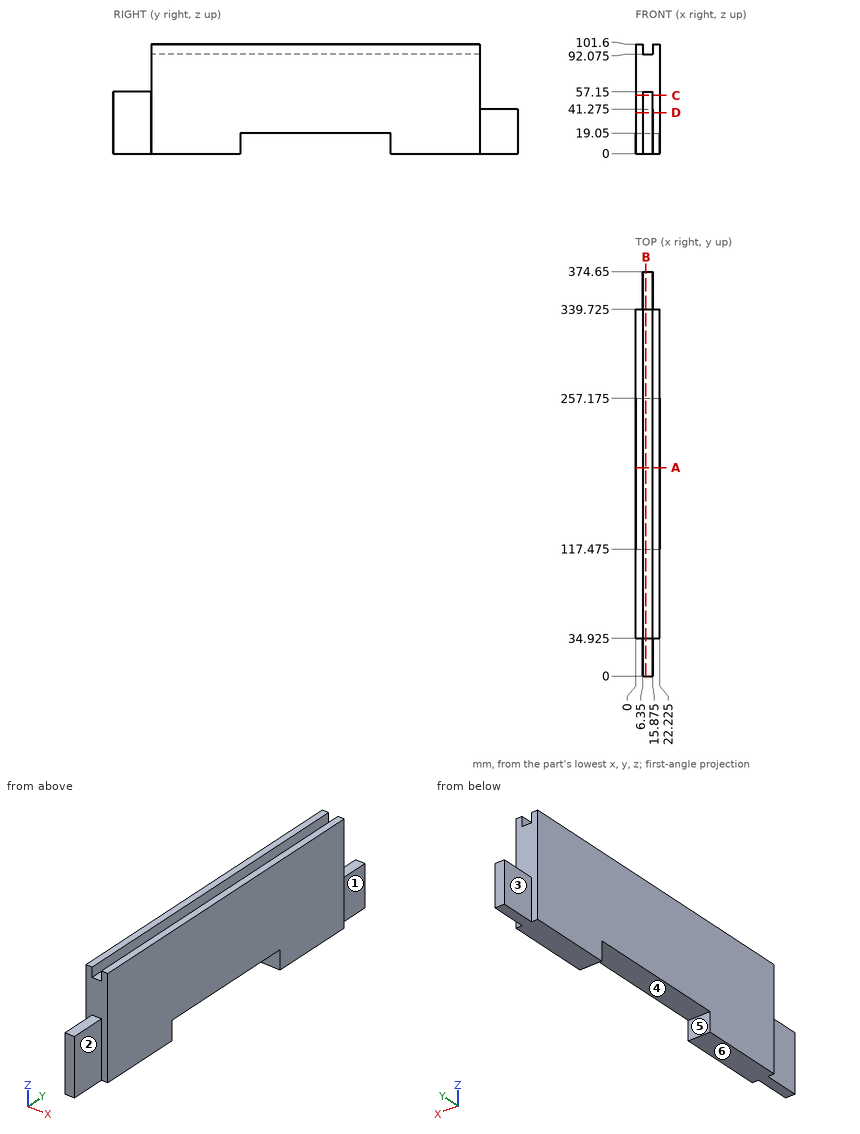
The figure shows three views and two pictorial views of one solid part (mm, origin at its lowest corner). Answer the questions. A direction names the side the tool comes from. Coordinates: 2 decimals unless noted, no trailing zeros. Order: outer loops, then holes, each group sorted by start corner. A loop starts at its lowest first (then second) coordinate and runs counter-clockwise, first axis right, second up.
Q1. A cutting plane is placed at C-C, the plane z = 54. Write down the section's boundary in (x, y) (3 decimals), and give its area (3 significant figures).
Q2. A cutting plane is placed at B-B, the plane x = 9.5. Write down the section's boundary in (y, z) (3 decimals).
Q3. A cutting plane is placed at D-D, the plane z = 38. Write down the section's boundary in (x, y) (3 decimals).
Q4. Given P1, Ø11, axis at x = 16, y = 198, coming from the -Z side; P2, Ø5, axis at x = 12, y = 250, coming from the +Z side (3 decimals); P3, Ø5, axis at x = 9.5, z = 79.5, coming from the +Y side (3 decimals), each flat-ended and moving along its own axis, determine where each tip first touches the part or whether it passes through.
Q5. Which of the six approach directions +Z, -Z, +X, -X, +Y, -Y give full straight-line access (tool end or side, diameter ignored) to the marked faces 1, 2, 3 and 4?
Q6. A cutting plane is placed at A-A, the plane y = 193. Write down the section's boundary in (x, z) (3 decimals), and give its area (3 significant figures).
Q7. Consider line 1 (Y direction, x = 9, z = 7) (3 decimals); line 2 (Y direction, x = 20.5, z = 4) (3 decimals); line 3 (Y direction, x = 21, z = 69.5) (3 decimals). Determine where each line is inside the solid, lowest interval first.
Q8. For a pull along Y with two mould halves and no side action, classify the marked faces 5 and 6 as pulls with the +Y half, pulls with the -Y half, needs draft (parallel to the pull), parting line crosses it, or undercut.
Answers follow:
1. outline: (0, 34.925) - (6.35, 34.925) - (6.35, 0) - (15.875, 0) - (15.875, 34.925) - (22.225, 34.925) - (22.225, 339.725) - (0, 339.725) - close
1. area: 7,110 mm2
2. outline: (0, 0) - (117.475, 0) - (117.475, 19.05) - (257.175, 19.05) - (257.175, 0) - (374.65, 0) - (374.65, 41.275) - (339.725, 41.275) - (339.725, 92.075) - (34.925, 92.075) - (34.925, 57.15) - (0, 57.15) - close
3. outline: (0, 34.925) - (6.35, 34.925) - (6.35, 0) - (15.875, 0) - (15.875, 34.925) - (22.225, 34.925) - (22.225, 339.725) - (15.875, 339.725) - (15.875, 374.65) - (6.35, 374.65) - (6.35, 339.725) - (0, 339.725) - close
4. P1: stops at z = 19.05
4. P2: stops at z = 92.075
4. P3: stops at y = 339.725
5. face 1: +Z, -Z, +X, +Y
5. face 2: +Z, -Z, +X, -Y
5. face 3: +Z, -Z, -X, +Y
5. face 4: -Z, +X, -X
6. outline: (0, 19.05) - (22.225, 19.05) - (22.225, 101.6) - (15.875, 101.6) - (15.875, 92.075) - (6.35, 92.075) - (6.35, 101.6) - (0, 101.6) - close
6. area: 1,740 mm2
7. line 1: y = 0 to 117.475, 257.175 to 374.65
7. line 2: y = 34.925 to 117.475, 257.175 to 339.725
7. line 3: y = 34.925 to 339.725
8. face 5: undercut
8. face 6: needs draft
